Can you work these out from the drawing? Everything is in mm from the part's minimum corner. A direction names the side the tool comes from. Round coordinates to 2 decimals unless told otherwise and drop trailing zeros. Write each loop counter-clockwise with the first axis right and the second up, starting at its lowest first coordinate (ties: lowest second). Pieces come first, ordered by that corner, then holes. Notation, with made-up numbers: (72, -9.75) -> (112, -9.75) arc R16 cw to (112, 0.25) -> close; hole circle Ø11 at (22.25, -18.75). An arc over 180 degrees is marked (long way). Write item = value, one per line. Start each with the question number.
1) If I drill on line 1 (Y direction, x = 21, z = 12.7); line 2 (X direction, y = 35.5, z = 25.5) (1 decimal); line 3 (Z direction, x = 17.5, y = 14), over which ranges is the centre line in solid material (lowest first)?
2) Thinking about a two-plate mould opening in Z: for the marked faces 1, 2 and 3, which applies, +Z half, -Z half, draft (parallel to the pull), parting line (faces both ways), or undercut?
3) Imagine slicing it at B-B, the plane x = 9. Please give me the cut outline in (y, z).
4) I'm going to push flat-ended pins straight in: pin 1 (5 mm diameter, centred on x = 35, y = 14, fed in from -Z); pin 2 (6 mm diameter, centred on y = 50.8, z = 12.7, fed in from -X); pin 3 (8.5 mm diameter, centred on y = 33, z = 18, fed in from +X). Where does each tip first touch, or does it pass through?
5) For the marked faces 4 and 5, which set-ups out of +Z, -Z, +X, -X, +Y, -Y let a thin tool reach every point of the face, with its end or its side?
6) Imagine slicing it at A-A, the plane y = 25.4. State how many separate pieces and enclosed holes the cut face has, then the cut area to 3 significant figures.
7) Imagine slicing it at C-C, the plane z = 38.1. Please give me the cut outline in (x, y), then the cut area to 3 significant figures.
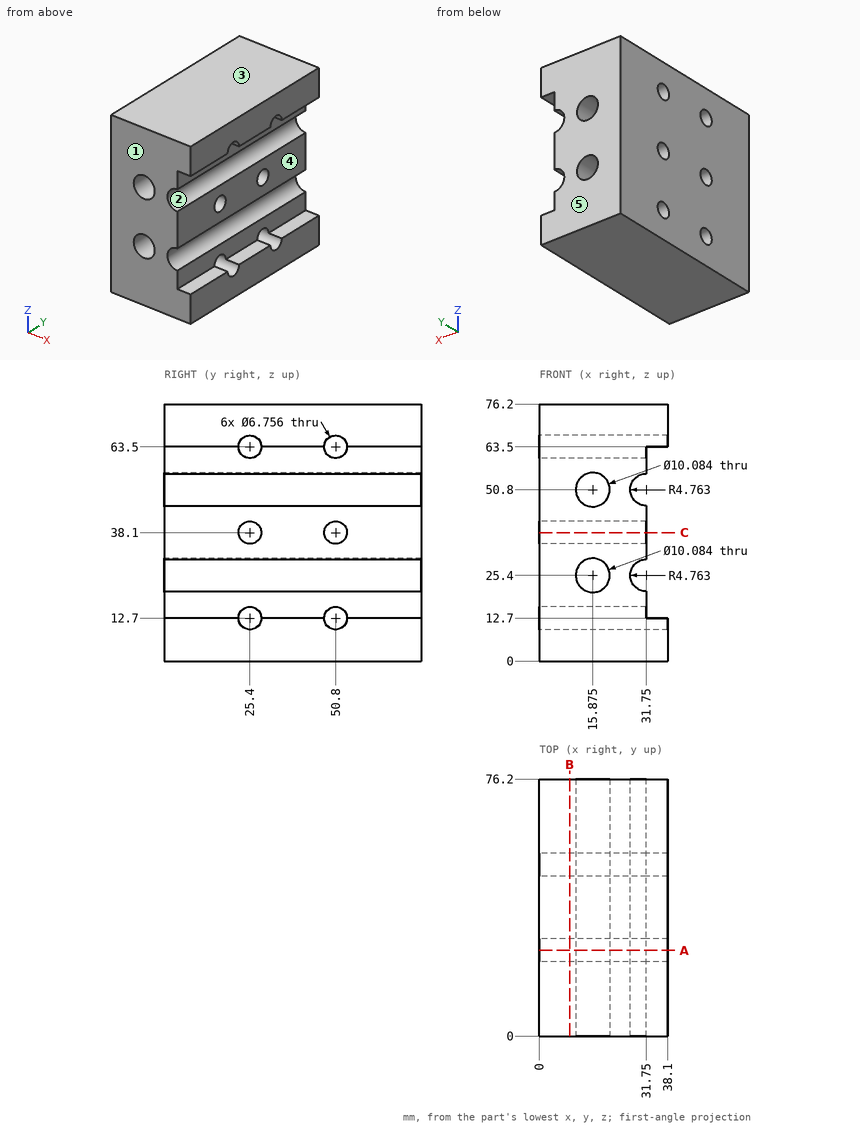
Reported:
q1.line_1 = 0 to 22.02, 28.78 to 47.42, 54.18 to 76.2
q1.line_2 = 0 to 10.8, 20.9 to 27
q1.line_3 = 0 to 20.63, 30.17 to 46.03, 55.57 to 76.2
q2.face_1 = draft
q2.face_2 = undercut
q2.face_3 = +Z half
q3.outline = (0, 0) -> (76.2, 0) -> (76.2, 76.2) -> (0, 76.2) -> close; hole circle Ø6.76 at (25.4, 12.7); hole circle Ø6.76 at (25.4, 38.1); hole circle Ø6.76 at (25.4, 63.5); hole circle Ø6.76 at (50.8, 12.7); hole circle Ø6.76 at (50.8, 38.1); hole circle Ø6.76 at (50.8, 63.5)
q4.pin_1 = 0
q4.pin_2 = through
q4.pin_3 = 31.75
q5.face_4 = +X, +Y, -Y
q5.face_5 = +Z, -Z, +X, -X, +Y
q6.separate_pieces = 4
q6.enclosed_holes = 2
q6.area = 1,660 mm²
q7.outline = (0, 0) -> (31.75, 0) -> (31.75, 22.02) -> (0, 22.02) -> close; (0, 28.78) -> (31.75, 28.78) -> (31.75, 47.42) -> (0, 47.42) -> close; (0, 54.18) -> (31.75, 54.18) -> (31.75, 76.2) -> (0, 76.2) -> close
q7.area = 1,990 mm²
